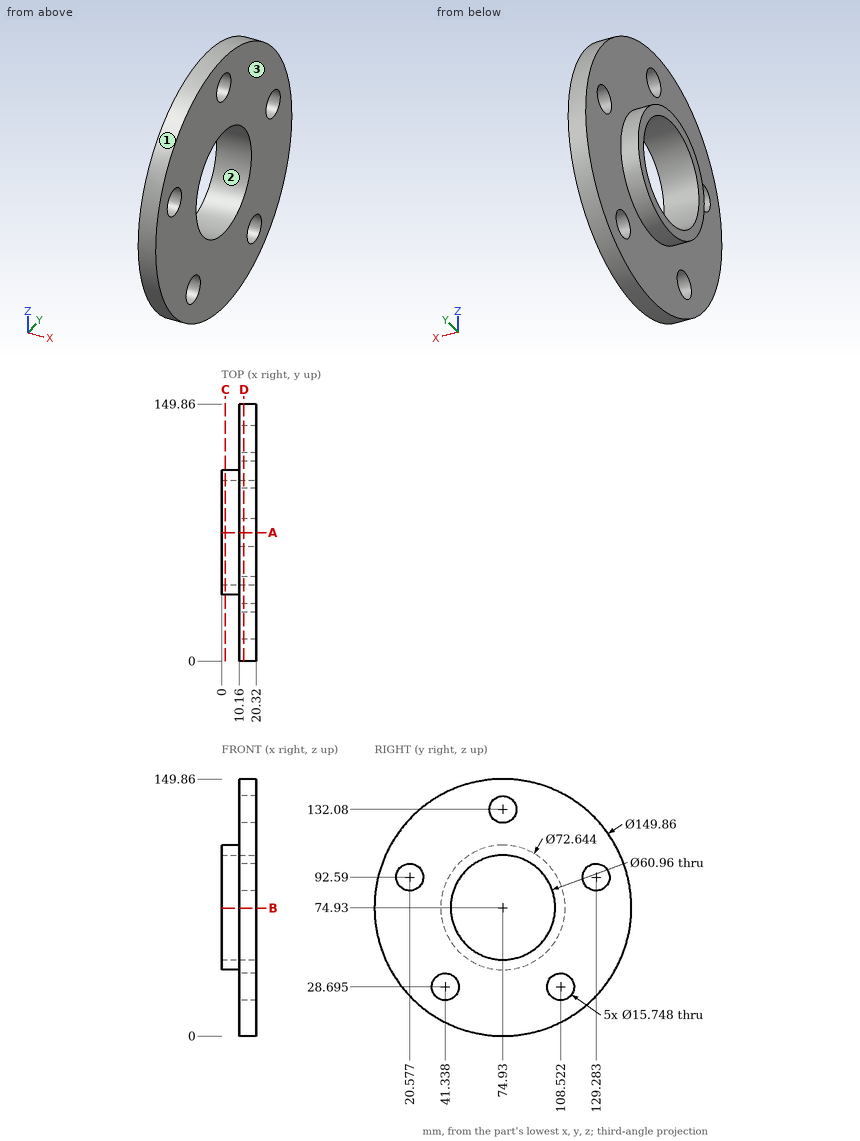
Input: dimensioned drawing with shaded views. Units: mm. Origin: part minimum x, y, z. Give positions to 0.01 mm unless a question says otherwise; leave off trailing zeros. Order: outer loops, then holes, each group sorted by start corner. A loop starts at its lowest first (then second) coordinate and runs counter-clockwise, first axis right, second up.
(1) Section query A-A (y = 74.93). Return the cut outline in (x, z).
(2) Contact query for flat-ended pins moving along their axis: P1, Ø20.5, axis at y = 129.28, z = 92.59, coming from the -X side; P2, Ø18, axis at y = 74.93, z = 132.08, coming from the +X side; P3, Ø6, axis at x = 18, z = 43.5, coming from the +Y side; P4, Ø12.5, axis at y = 108.52, z = 28.69, coming from the +X side. Output: stop coordinate, or through.
(3) Section query B-B (z = 74.5). Return the cut outline in (x, y).
(4) Section query D-D (x = 13). State how many separate pieces and enclosed holes the cut face has, plus the area to 3 significant figures.
(5) Pull-direction query (Y, two-part tool) for the marked faces 1, 2 and 3; classes: +Y half, -Y half, draft (parallel to the pull), parting line (faces both ways), or undercut.
(6) Section query C-C (x = 2.25). Return the cut outline in (y, z).
(7) Material intervals for line 1 along Z through (x, y) = (17.75, 74.93); line 2 along Y through (x, z) = (13, 74.93); line 3 along X through (y, z) = (93, 116.5), sorted ascending.
Outcome:
1. outline: (0, 38.61) - (10.16, 38.61) - (10.16, 0) - (20.32, 0) - (20.32, 44.45) - (0, 44.45) - close; (0, 105.41) - (20.32, 105.41) - (20.32, 124.21) - (10.16, 124.21) - (10.16, 111.25) - (0, 111.25) - close; (10.16, 139.95) - (20.32, 139.95) - (20.32, 149.86) - (10.16, 149.86) - close
2. P1: stops at x = 10.16
2. P2: stops at x = 20.32
2. P3: stops at y = 144.26
2. P4: passes through
3. outline: (0, 38.61) - (10.16, 38.61) - (10.16, 0) - (20.32, 0) - (20.32, 44.45) - (0, 44.45) - close; (0, 105.41) - (20.32, 105.41) - (20.32, 149.86) - (10.16, 149.86) - (10.16, 111.25) - (0, 111.25) - close
4. separate pieces: 1
4. enclosed holes: 6
4. area: 13,700 mm2
5. face 1: parting line
5. face 2: undercut
5. face 3: draft
6. outline: circle Ø72.64 at (74.93, 74.93); hole circle Ø60.96 at (74.93, 74.93)
7. line 1: z = 0 to 44.45, 105.41 to 124.21, 139.95 to 149.86
7. line 2: y = 0 to 44.45, 105.41 to 149.86
7. line 3: x = 10.16 to 20.32
